Design review of the part built by this model. Coordinates are the model's own, in mm. Face numbers are marked on the shaded views. Round coordinates to 2 decimals unless told otherwise and drop trailing zeros. Write each loop counter-clockwise with the first axis right and the second up, starting at its lowest first coordinate (ties: lowest second). Pieces come first, ordered by that corner, then holes. Notation, with made-up numbers: (6.5, 65.25) -> (46.5, 65.25) arc R24 ccw to (46.5, 82.25) -> close; hole circle Ø4 at (12, -13). An arc over 180 degrees is marked (long way). Write item = value, one per line. Start each with the question number.
Item 1: To check wall thickness, follow L1, parallel to Y at x = -29.5, z = 2; L2, parallel to Y at x = 32, z = 1.05; L3, parallel to Z at x = 1, y = -32. State the ranges of each line that lie inside material, in increasing order.
Item 2: Add section A-A, the plane y = -30. State the section outline as (x, z) points.
Item 3: Add section B-B, the plane x = -3. State the section outline as (y, z) points.
Item 4: Add section D-D, the plane y = 5. State the section outline as (x, z) points.
Item 5: For pin 1 Ø5.5 at (x, z) = (-17.5, 17) entering from -Y; pin 2 Ø1 at (y, z) = (-25, 5.5) entering from +X; pin 3 Ø1.5 at (x, z) = (-20, 5) entering from +Y, all flat-tipped, find the tip position at first contact; note any pin that passes through.
Item 6: Add section C-C, the plane z = 6. State the section outline as (x, y) points.
Item 7: Mouldability with a two-part tool opening along X and no side actions: class the marked faces 1, 2 and 3 as released by +X, released by -X, zero draft, split by the parting line, or undercut.
Solid Edge part; units mm, degrees
sketch "Sketch1" plane through (0, 0, 0) normal (0, 0, 1) x (1, 0, 0)
  line L0 (-40, -40) -> (40, -40)
  line L1 (40, -40) -> (40, 40)
  line L2 (40, 40) -> (-40, 40)
  line L3 (-40, 40) -> (-40, -40)
extrude "Protrusion1" add sketch "Sketch1" along normal blind 4
sketch "Sketch2" plane through (0, 0, 4) normal (0, 0, 1) x (1, 0, 0)
  line L0 (-14.05, -37) -> (-14.05, -24)
  line L1 (-14.05, -24) -> (-21.05, -24)
  line L2 (-21.05, -24) -> (-21.05, -37)
  line L3 (-21.05, -37) -> (-14.05, -37)
  line L4 (14.05, -24) -> (14.05, -37)
  line L5 (14.05, -37) -> (21.05, -37)
  line L6 (21.05, -37) -> (21.05, -24)
  line L7 (21.05, -24) -> (14.05, -24)
extrude "Extrusionsausprägung_2" add sketch "Sketch2" along normal blind 18
sketch "Sketch3" plane through (-18.15, -37, 13) normal (0, -1, 0) x (1, 0, 0)
  circle A0 centre (0.6, 6) radius 1.5
extrude "Extrusionsausschnitt_1" cut sketch "Sketch3" against normal blind 38.6
sketch "Sketch4" plane through (18.15, -37, 13) normal (0, -1, 0) x (1, 0, 0)
  circle A0 centre (-0.6, 5) radius 1.5
extrude "Extrusionsausschnitt_2" cut sketch "Sketch4" against normal blind 51.3
fillet "Verrundung_1" radius 2 4 edges at (-21.05, -30.5, 22) (-14.05, -30.5, 22) (14.05, -30.5, 22) (21.05, -30.5, 22)
sketch "Sketch5" plane through (0, 0, 4) normal (0, 0, 1) x (1, 0, 0)
  circle A0 centre (32, -30) radius 2.25
  circle A1 centre (29, 5) radius 1
  circle A2 centre (29, 34) radius 1
  circle A3 centre (3, 5) radius 1
  circle A4 centre (-3, 5) radius 1
  circle A5 centre (3, 34) radius 1
  circle A6 centre (-3, 34) radius 1
  circle A7 centre (-29, 34) radius 1
  circle A8 centre (-29, 5) radius 1
  circle A9 centre (-32, -30) radius 2.25
extrude "Cutout1" cut sketch "Sketch5" against normal blind 112.1
fillet "Verrundung_2" radius 4 4 edges at (-40, 40, 2) (-40, -40, 2) (40, -40, 2) (40, 40, 2)
fillet "Verrundung_3" radius 1 8 edges at (0, 40, 4) (-38.8284, 38.8284, 4) (-40, 0, 4) (-38.8284, -38.8284, 4) (0, -40, 4) (38.8284, -38.8284, 4) (40, 0, 4) (38.8284, 38.8284, 4)
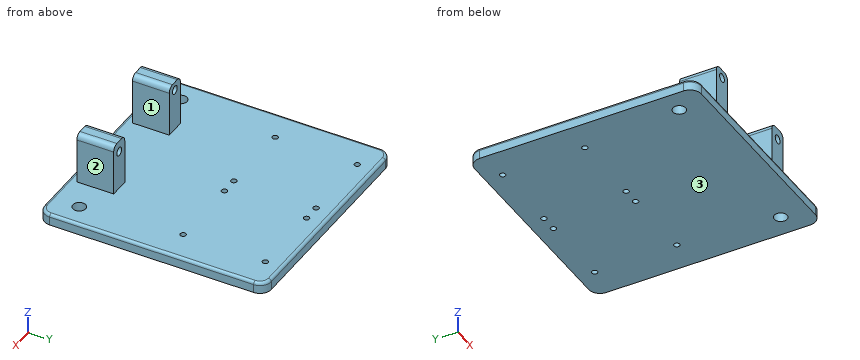
Result set:
q1.L1 = -40 to 4.13, 5.87 to 33.13, 34.87 to 40
q1.L2 = -40 to -32.25, -27.75 to 40
q1.L3 = 0 to 4
q2.outline = (-40, 0) -> (-34.25, 0) -> (-34.25, 4) -> (-39, 4) arc R1 ccw to (-40, 3) -> close; (-29.75, 0) -> (29.75, 0) -> (29.75, 4) -> (21.05, 4) -> (21.05, 20) arc R2 ccw to (19.05, 22) -> (16.05, 22) arc R2 ccw to (14.05, 20) -> (14.05, 4) -> (-14.05, 4) -> (-14.05, 20) arc R2 ccw to (-16.05, 22) -> (-19.05, 22) arc R2 ccw to (-21.05, 20) -> (-21.05, 4) -> (-29.75, 4) -> close; (34.25, 0) -> (40, 0) -> (40, 3) arc R1 ccw to (39, 4) -> (34.25, 4) -> close; hole circle Ø3 at (-17.55, 19); hole circle Ø3 at (17.55, 18)
q3.outline = (-40, 0) -> (4, 0) -> (4, 4) -> (-39, 4) arc R1 ccw to (-40, 3) -> close; (6, 0) -> (33, 0) -> (33, 4) -> (6, 4) -> close; (35, 0) -> (40, 0) -> (40, 3) arc R1 ccw to (39, 4) -> (35, 4) -> close
q4.outline = (-40, 0) -> (-30, 0) -> (-30, 4) -> (-39, 4) arc R1 ccw to (-40, 3) -> close; (-28, 0) -> (-4, 0) -> (-4, 4) -> (-28, 4) -> close; (-2, 0) -> (2, 0) -> (2, 4) -> (-2, 4) -> close; (4, 0) -> (28, 0) -> (28, 4) -> (4, 4) -> close; (30, 0) -> (40, 0) -> (40, 3) arc R1 ccw to (39, 4) -> (30, 4) -> close
q5.pin_1 = -37
q5.pin_2 = 21.05
q5.pin_3 = -24
q6.outline = (-21.05, -37) -> (-14.05, -37) -> (-14.05, -24) -> (-21.05, -24) -> close; (14.05, -37) -> (21.05, -37) -> (21.05, -24) -> (14.05, -24) -> close
q7.face_1 = undercut
q7.face_2 = released by +X
q7.face_3 = zero draft
